from build123d import *

# Parameters (mm, degrees)
SKETCH1_W           = 24
SKETCH1_H           = 19
SKETCH1_W_2         = 20
SKETCH1_H_2         = 15
BOSS_EXTRUDE1_DEPTH = 13
SKETCH2_W           = 13.396276459
SKETCH2_H           = 6.003539649
SKETCH2_R           = 2.05
SKETCH2_W_2         = 12.603723541
SKETCH2_H_2         = 6
BOSS_EXTRUDE2_DEPTH = 5
SKETCH4_W           = 3
SKETCH4_H           = 20
BOSS_EXTRUDE3_DEPTH = 2
SKETCH5_W           = 2
SKETCH5_H           = 3
BOSS_EXTRUDE4_DEPTH = 4
SKETCH6_W           = 2
SKETCH6_H           = 3
BOSS_EXTRUDE5_DEPTH = 4
CHAMFER1_SIZE       = 1
CHAMFER1_SIZE2      = 1.732050808
FILLET1_R           = 2
CHAMFER2_SIZE       = 1
CHAMFER2_SIZE2      = 1.732050808


with BuildPart() as part:
    # Sketch1 → Boss-Extrude1 (new body)
    with BuildSketch(Plane(origin=(0, 0, 0), x_dir=(0, 0, -1), z_dir=(1, 0, 0))):
        with Locations((10, -7.5)):
            Rectangle(SKETCH1_W, SKETCH1_H)
        with Locations((10, -7.5)):
            Rectangle(SKETCH1_W_2, SKETCH1_H_2, mode=Mode.SUBTRACT)
    extrude(amount=BOSS_EXTRUDE1_DEPTH)

    # Sketch2 → Boss-Extrude2 (add)
    # profile 1 of 2: a face of its own
    with BuildSketch(Plane.ZY):
        with Locations((-28.698138229, -13.998230176)):
            Rectangle(SKETCH2_W, SKETCH2_H)
        with Locations((-33, -13.998230176)):
            Circle(SKETCH2_R, mode=Mode.SUBTRACT)
    # profile 2 of 2: a face of its own
    with BuildSketch(Plane.ZY):
        with Locations((8.301861771, -14)):
            Rectangle(SKETCH2_W_2, SKETCH2_H_2)
        with Locations((11.299999965, -14)):
            Circle(SKETCH2_R, mode=Mode.SUBTRACT)
    extrude(amount=-BOSS_EXTRUDE2_DEPTH)

    # Sketch4 → Boss-Extrude3 (add)
    with BuildSketch(Plane.XZ):
        with Locations((1.5, -10)):
            Rectangle(SKETCH4_W, SKETCH4_H)
    extrude(amount=BOSS_EXTRUDE3_DEPTH)

    # Sketch5 → Boss-Extrude4 (add)
    with BuildSketch(Plane(origin=(0, 2, 0), x_dir=(1, 0, 0), z_dir=(0, 1, 0))):
        with Locations((10, 10)):
            Rectangle(SKETCH5_W, SKETCH5_H)
    extrude(amount=BOSS_EXTRUDE4_DEPTH)

    # Sketch6 → Boss-Extrude5 (add)
    with BuildSketch(Plane.XZ.offset(17)):
        with Locations((10, -10)):
            Rectangle(SKETCH6_W, SKETCH6_H)
    extrude(amount=BOSS_EXTRUDE5_DEPTH)

    # Chamfer1
    chamfer1_edges = [part.edges().sort_by_distance(p)[0] for p in [
        (10, 2, -8.5),
        (11, 2, -10),
        (10, 2, -11.5),
    ]]
    chamfer1_side = [part.faces().sort_by_distance(p)[0] for p in [
        (6.431372549, 2, -10),
    ]]
    chamfer(chamfer1_edges, length=CHAMFER1_SIZE, length2=CHAMFER1_SIZE2, reference=chamfer1_side[0])

    # Fillet1
    fillet1_edges = [part.edges().sort_by_distance(p)[0] for p in [
        (6.5, 2, 2),
        (6.5, 2, -22),
        (9, -17, -22),
        (9, -17, 2),
    ]]
    fillet(fillet1_edges, radius=FILLET1_R)

    # Chamfer2
    chamfer2_edges = [part.edges().sort_by_distance(p)[0] for p in [
        (10, -17, -11.5),
        (11, -17, -10),
        (10, -17, -8.5),
    ]]
    chamfer2_side = [part.faces().sort_by_distance(p)[0] for p in [
        (4.962871287, -17, -10.245220581),
    ]]
    chamfer(chamfer2_edges, length=CHAMFER2_SIZE, length2=CHAMFER2_SIZE2, reference=chamfer2_side[0])


solid = part.part
Here's how the part is built. I have some questions about the finished solid (model axes, mm). A direction names the side the tool comes from. Give positions to 0.01 mm unless a question says otherwise; leave off trailing zeros. Order: outer loops, then holes, each group sorted by start corner. A loop starts at its lowest first (then second) coordinate and runs counter-clockwise, first axis right, second up. Notation, with made-up numbers: M 41,-20 L 67,-20 A27 cw 67,-3 Z; hole C 81.25,50 d11. An arc over 180 degrees is marked long. Answer as a JSON object with one key per item and string values. Group by question number.
1) Suppose I cut it at C-C, the plane x = 10. Write out the boundary of the cut face in (y, z).
2) Please list where these lines run through material, in increasing order: L1, parallel to Z at x = 11.5, y = -9.5; L2, parallel to Y at x = 1.15, z = -33; L3, parallel to Z at x = 4.5, y = -11.5. Write a range as [from, to].
3) We'd pull the mould along Y, two halves only. Please class faces 1 (the flat face through (13, -16, -10)), 2 (the cylindrical face through (6.59, 1.43, 1.4)), 3 (the cylindrical face through (9.06, -16.43, -21.4)), 4 (the cylindrical face through (2.465, -15.246, -34.627)): pulls with the +Y half, pulls with the -Y half, needs draft (parallel to the pull), parting line crosses it, or undercut.
4) Suppose I cut it at B-B, the plane y = -7. Write out the boundary of the cut face in (x, z), plus the area to 3 significant figures.
5) Suppose I cut it at D-D, the plane x = 2.25. Write out the boundary of the cut face in (y, z), plus the area to 3 significant figures.
6) I'm going to push flat-ended pins straight in: pin 1 Ø2 at (x, y) = (10.5, 4.5) entering from +Z; pin 2 Ø4 at (x, y) = (8.5, -4.5) entering from -Z; pin 3 Ø5 at (x, z) = (6.5, -26.5) entering from -Y; pin 4 Ø8 at (y, z) = (-6.5, 3.5) entering from +X. Where does each tip first touch, or does it pass through?
7) On a 3-axis mill with a long thin cutter (end or side, diameter ignored), from which of +Z, -Z, +X, -X, +Y, -Y can I reach the whole of each face in a straight line? I mean faces 5 (the flat face through (10, 5, -11.5)), 6 (the flat face through (11, 5, -10)), 7 (the flat face through (9, -19, -10)). Say none if no direction works.
8) Suppose I cut it at A-A, the plane z = 11.3. Write out the boundary of the cut face in (x, y), plus the area to 3 significant figures.
Results found:
{
 "1": {"outline": "M -21,-11.5 L -18.73,-11.5 L -17,-12.5 L -17,-20 A2 ccw -15,-22 L 0,-22 A2 ccw 2,-20 L 2,-12.5 L 3.73,-11.5 L 6,-11.5 L 6,-8.5 L 3.73,-8.5 L 2,-7.5 L 2,0 A2 ccw 0,2 L -15,2 A2 ccw -17,0 L -17,-7.5 L -18.73,-8.5 L -21,-8.5 Z; hole M -15,-20 L 0,-20 L 0,0 L -15,0 Z"},
 "2": {"L1": "[-22, -20], [0, 2]", "L2": "[-17, -16.05], [-11.95, -11]", "L3": "[-35.4, -20], [0, 14.6]"},
 "3": {"face 1": "needs draft", "face 2": "pulls with the +Y half", "face 3": "pulls with the -Y half", "face 4": "undercut"},
 "4": {"outline": "M 0,-22 L 13,-22 L 13,-20 L 0,-20 Z; M 0,0 L 13,0 L 13,2 L 0,2 Z", "area": "52.0 mm²"},
 "5": {"outline": "M -17,-35.4 L -11,-35.4 L -11,-22 L 0,-22 A2 ccw 2,-20 L 2,0 A2 ccw 0,2 L -11,2 L -11,14.6 L -17,14.6 Z; hole C -14,-33 d4.1; hole C -14,11.3 d4.1; hole M -15,-20 L -2,-20 L -2,0 L -15,0 Z", "area": "324 mm²"},
 "6": {"pin 1": "z = -8.37", "pin 2": "z = -22", "pin 3": "y = -17", "pin 4": "x = 13"},
 "7": {"face 5": "-Z, +X, -X, +Y", "face 6": "+Z, -Z, +X, +Y", "face 7": "+Z, -Z, -X, -Y"},
 "8": {"outline": "M 0,-17 L 5,-17 L 5,-16.05 L 0,-16.05 Z; M 0,-11.95 L 5,-11.95 L 5,-11 L 0,-11 Z", "area": "9.50 mm²"}
}
